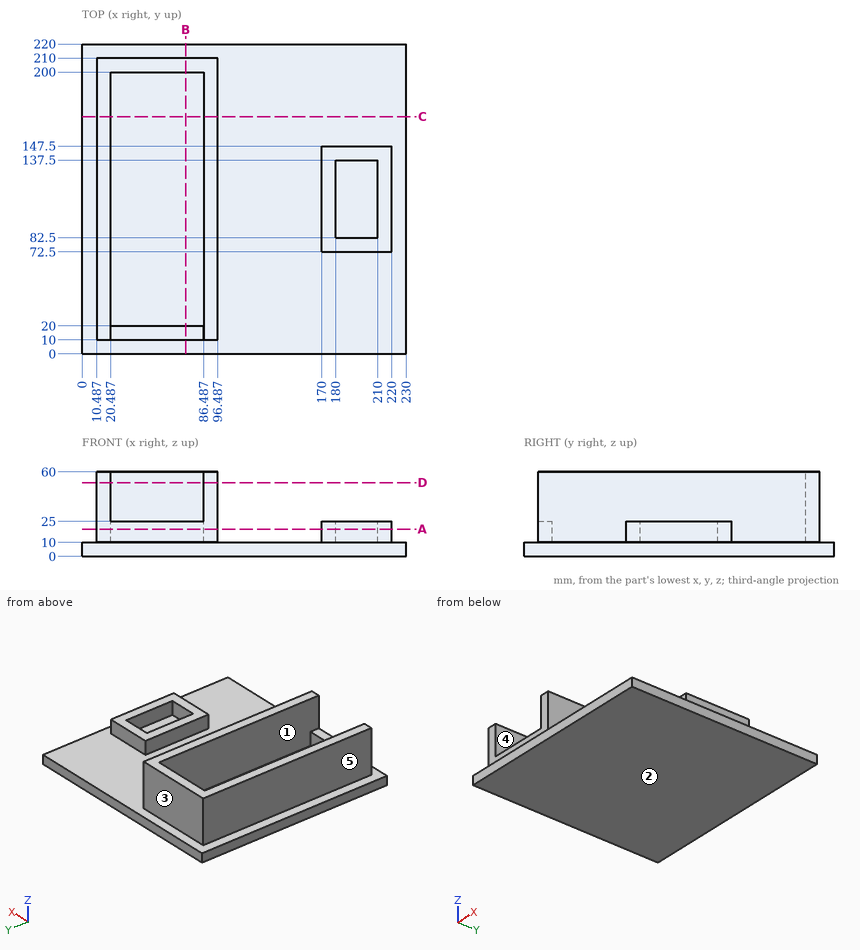
Verification items for this drawing (mm, ordinates from the low corner). A direction names the side the tool comes from. Round coordinates to 2 decimals unless told otherwise and drop trailing zeros. Loops run counter-clockwise (first coordinate to the right, second up) from the corner with the lowest first, then second, coordinate; pieces in that order, holes last. Notation, with made-up numbers: (-1.75, 89.25) -> (19.25, 89.25) arc R25 cw to (19.25, 119.25) -> close; hole circle Ø4 at (35, -27). An arc over 180 degrees is marked (long way). Write item = value, one per line. Start each with the question number.
1) Sectioned sample at D-D, the plane z = 52.5. Record the cut outline in (x, y), plus the area to 3 significant figures.
2) Sectioned sample at A-A, the plane z = 19.5. Record the cut outline in (x, y), plus the area to 3 significant figures.
3) Gauge pin test, flat ends, axial feed: pin 1 Ø3 at (x, z) = (69, 35) entering from +Y; pin 2 Ø10 at (x, y) = (48.5, 123.5) entering from +Z; pin 3 Ø6 at (y, z) = (40.5, 27) entering from +X. Record the tip position at first contact, or that the pin passes through.
4) Sectioned sample at B-B, the plane x = 73.5. Record the cut outline in (y, z), plus the area to 3 significant figures.
5) Release check for a two-part mould opening along X. For the marked faces 3, 4 and 5 record: released by +X, released by -X, zero draft, split by the parting line, or undercut.
6) Thickness scan on probe 1 along X at (y, z) = (122, 49); probe 2 along Y at (x, z) = (86, 30.5); probe 3 along Z at (x, y) = (109, 180.5). Record the ranges inside material, lowest first.
7) Sectioned sample at C-C, the plane y = 168.5. Record the cut outline in (x, z), plus the area to 3 significant figures.
8) Set-up check for the marked faces 1 and 2: record each of +Z, -Z, +X, -X, +Y, -Y from which the full face is reachable in a straight line by a thin tool's end or side.
Results are:
q1.outline = (10.49, 10) -> (20.49, 10) -> (20.49, 200) -> (86.49, 200) -> (86.49, 10) -> (96.49, 10) -> (96.49, 210) -> (10.49, 210) -> close
q1.area = 4,660 mm^2
q2.outline = (10.49, 10) -> (96.49, 10) -> (96.49, 210) -> (10.49, 210) -> close; (170, 72.5) -> (220, 72.5) -> (220, 147.5) -> (170, 147.5) -> close; hole (20.49, 20) -> (86.49, 20) -> (86.49, 200) -> (20.49, 200) -> close; hole (180, 82.5) -> (210, 82.5) -> (210, 137.5) -> (180, 137.5) -> close
q2.area = 7,420 mm^2
q3.pin_1 = 210
q3.pin_2 = 10
q3.pin_3 = 96.49
q4.outline = (0, 0) -> (220, 0) -> (220, 10) -> (210, 10) -> (210, 60) -> (200, 60) -> (200, 10) -> (20, 10) -> (20, 25) -> (10, 25) -> (10, 10) -> (0, 10) -> close
q4.area = 2,850 mm^2
q5.face_3 = zero draft
q5.face_4 = undercut
q5.face_5 = released by -X
q6.probe_1 = 10.49 to 20.49, 86.49 to 96.49
q6.probe_2 = 200 to 210
q6.probe_3 = 0 to 10
q7.outline = (0, 0) -> (230, 0) -> (230, 10) -> (96.49, 10) -> (96.49, 60) -> (86.49, 60) -> (86.49, 10) -> (20.49, 10) -> (20.49, 60) -> (10.49, 60) -> (10.49, 10) -> (0, 10) -> close
q7.area = 3,300 mm^2
q8.face_1 = +Z
q8.face_2 = -Z, +X, -X, +Y, -Y
